For this review, take the finished solid that the model builds, in its own axes (mm). A direction names the side the tool comes from. Coordinates: 2 decimals unless noted, no trailing zeros. Order: outer loops, then holes, each group sorted by start corner. A loop starts at its lowest first (then second) coordinate and runs counter-clockwise, first axis right, second up.
from build123d import *

# Parameters (mm, degrees)
SKETCH1_W           = 70
SKETCH1_H           = 100
SKETCH1_W_2         = 10
SKETCH1_H_2         = 3
BOSS_EXTRUDE1_DEPTH = 3
SKETCH2_W           = 10
SKETCH2_H           = 3
CUT_EXTRUDE1_DEPTH  = 64.584589328
SKETCH3_R           = 15
CUT_EXTRUDE2_DEPTH  = 64.584589328


with BuildPart() as part:
    # Sketch1 → Boss-Extrude1 (new body)
    with BuildSketch(Plane.XY):
        Rectangle(SKETCH1_W, SKETCH1_H)
        with Locations((21.5, -51.5)):
            Rectangle(SKETCH1_W_2, SKETCH1_H_2)
        with Locations((1.5, -51.5)):
            Rectangle(SKETCH1_W_2, SKETCH1_H_2)
        with Locations((-18.5, -51.5)):
            Rectangle(SKETCH1_W_2, SKETCH1_H_2)
    extrude(amount=BOSS_EXTRUDE1_DEPTH)

    # Sketch2 → Cut-Extrude1 (cut, through all)
    with BuildSketch(Plane.XY.offset(3)):
        with Locations((-20, 48.5)):
            Rectangle(SKETCH2_W, SKETCH2_H)
        with Locations((0, 48.5)):
            Rectangle(SKETCH2_W, SKETCH2_H)
        with Locations((20, 48.5)):
            Rectangle(SKETCH2_W, SKETCH2_H)
    extrude(amount=-CUT_EXTRUDE1_DEPTH, mode=Mode.SUBTRACT)

    # Sketch3 → Cut-Extrude2 (cut, through all)
    with BuildSketch(Plane.XY.offset(3)):
        with Locations((0, 22)):
            Circle(SKETCH3_R)
    extrude(amount=-CUT_EXTRUDE2_DEPTH, mode=Mode.SUBTRACT)


solid = part.part
1. Clearance check with flat-ended pins moving along their axes: pin 1 Ø1.5 at (x, z) = (19, 1.5) entering from +Y; pin 2 Ø1.5 at (x, z) = (14, 2) entering from -Y; pin 3 Ø0.9 at (y, z) = (-51, 1.5) entering from -X. State where each tip first meets the part, or that it passes through.
Answer below:
pin 1: stops at y = 47
pin 2: stops at y = -50
pin 3: stops at x = -23.5
2. To check wall thickness, follow L1, parallel to Y at x = 0, z = 1; L2, parallel to Y at x = 13, z = 1.75; L3, parallel to X at y = 35, z = 2.25. State the ranges of each line that lie inside material, in increasing order.
Answer below:
L1: y = -53 to 7, 37 to 47
L2: y = -50 to 14.52, 29.48 to 50
L3: x = -35 to -7.48, 7.48 to 35
3. Take a section at C-C, the plane x = 0. Give the boundary of the cut face in (y, z).
Answer below:
outline: (-53, 0) - (7, 0) - (7, 3) - (-53, 3) - close; (37, 0) - (47, 0) - (47, 3) - (37, 3) - close
4. Take a section at A-A, the plane y = 22. Give the boundary of the cut face in (x, z).
Answer below:
outline: (-35, 0) - (-15, 0) - (-15, 3) - (-35, 3) - close; (15, 0) - (35, 0) - (35, 3) - (15, 3) - close
5. The part is to be moulded in two halves that separate along X. For faces 4 (the face through (1, -53, 1)), 5 (the face through (-13.5, -52, 1)), 6 (the face through (15, 48, 2)), 7 (the face through (-35, -1, 1)), say which applies: +X half, -X half, draft (parallel to the pull), parting line (faces both ways), or undercut.
Answer below:
face 4: draft
face 5: undercut
face 6: undercut
face 7: -X half
6. Take a section at D-D, the plane x = -26. Give the boundary of the cut face in (y, z).
Answer below:
outline: (-50, 0) - (50, 0) - (50, 3) - (-50, 3) - close
7. Machinability: for faces 1 (the face through (-15, 48, 2)), 2 (the face through (31, -50, 1)), 3 (the face through (11, -50, 1)), which of the approach directions +Z, -Z, +X, -X, +Y, -Y give a long, thin tool a straight path to every point of the face, cutting with its end or side? Answer none if there is none.
Answer below:
face 1: +Z, -Z, +Y
face 2: +Z, -Z, +X, -Y
face 3: +Z, -Z, -Y
